Geometry: final body of the model. Coordinates: model frame, mm. A direction names the side the tool comes from. Round coordinates to 2 decimals unless told otherwise and drop trailing zeros. Loops run counter-clockwise (first coordinate to the right, second up) from the corner with the lowest first, then second, coordinate; pieces in that order, holes last. Notation, with made-up numbers: M 50,-1 L 69,-1 A32 ccw 69,26 Z; hole C 39.25,-18 d11. An arc over 180 degrees is marked long. Answer as a JSON object with one key per item and string values.
from build123d import *

# Parameters (mm, degrees)
AUFSATZ_LINEAR_AUSTRAGEN1_DEPTH = 50
SKIZZE2_R                       = 87.5
SKIZZE2_R_2                     = 35
AUFSATZ_LINEAR_AUSTRAGEN2_DEPTH = 50
SCHNITT_LINEAR_AUSTRAGEN1_DEPTH = 50


with BuildPart() as part:
    # Skizze1 → Aufsatz-Linear austragen1 (new body)
    with BuildSketch(Plane.XY):
        Polygon((0, 2300), (50, 2300), (475, 1237.5), (900, 2300), (950, 2300), (950, 2250), (510, 1150), (950, 50), (950, 0), (900, 0), (475, 1062.5), (50, 0), (0, 0), (0, 50), (440, 1150), (0, 2250), align=None)
    extrude(amount=AUFSATZ_LINEAR_AUSTRAGEN1_DEPTH)

    # Skizze2 → Aufsatz-Linear austragen2 (add)
    with BuildSketch(Plane.XY.offset(50)):
        with Locations((475, 1150)):
            Circle(SKIZZE2_R)
        with Locations((475, 1150)):
            Circle(SKIZZE2_R_2, mode=Mode.SUBTRACT)
    extrude(amount=-AUFSATZ_LINEAR_AUSTRAGEN2_DEPTH)

    # Skizze4 → Schnitt-Linear austragen1 (cut)
    with BuildSketch(Plane.XY.offset(50)):
        with BuildLine():
            ThreePointArc((512.5, 1150), (501.516504294, 1176.516504294), (475, 1187.5))
            Line((475, 1187.5), (475, 1112.5))
            ThreePointArc((475, 1112.5), (501.516504294, 1123.483495706), (512.5, 1150))
        make_face()
        with BuildLine():
            Line((475, 1112.5), (475, 1187.5))
            ThreePointArc((475, 1187.5), (437.5, 1150), (475, 1112.5))
        make_face()
    extrude(amount=-SCHNITT_LINEAR_AUSTRAGEN1_DEPTH, mode=Mode.SUBTRACT)


solid = part.part
1) Pin query (flat end, axial travel): P1, Ø1.5, axis at x = 240.5, z = 32.5, coming from the -Y side (3 decimals); P2, Ø5, axis at y = 467, z = 22.5, coming from the -X side; P3, Ø8, axis at y = 1826.5, z = 26, coming from the -X side. Return the tip coordinate at first contact, or that it passes through.
Results:
{"P1": "y = 474.375", "P2": "x = 165.8", "P3": "x = 167.8"}
2) Section query C-C (z = 26). Return the cut outline in (x, y), and give its area (3 significant figures).
Results:
{"outline": "M 0,0 L 50,0 L 475,1062.5 L 900,0 L 950,0 L 950,50 L 535.34,1086.64 A87.5 ccw 535.34,1213.36 L 950,2250 L 950,2300 L 900,2300 L 475,1237.5 L 50,2300 L 0,2300 L 0,2250 L 414.66,1213.36 A87.5 ccw 414.66,1086.64 L 0,50 Z; hole C 475,1150 d75", "area": "317,000 mm2"}
3) Reachability of faces 4 (the flat face through (745.575, 1738.937, 24.65)), 5 (the flat face through (690.475, 523.813, 24.65)), 6 (the flat face through (204.425, 561.063, 24.65)), 7 (the flat face through (950, 2275, 25)), 8 (the flat face through (437.6, 1155.4, 0)) from +Z, -Z, +X, -X, +Y, -Y: full face, straight path, thin tool, end or side. Return the list, or none.
Results:
{"face 4": "+Z, -Z, +X", "face 5": "+Z, -Z, -Y", "face 6": "+Z, -Z, -X", "face 7": "+Z, -Z, +X, +Y, -Y", "face 8": "-Z, +X, -X, +Y, -Y"}
4) Section query A-A (x = 824.5). Return the cut outline in (y, z).
Results:
{"outline": "M 188.75,0 L 363.75,0 L 363.75,50 L 188.75,50 Z; M 1936.25,0 L 2111.25,0 L 2111.25,50 L 1936.25,50 Z"}
5) Section query B-B (y = 316.5). Return the cut outline in (x, z).
Results:
{"outline": "M 106.6,0 L 176.6,0 L 176.6,50 L 106.6,50 Z; M 773.4,0 L 843.4,0 L 843.4,50 L 773.4,50 Z"}
6) Pull-direction query (Y, two-part tool) for faces 1 (the flat face through (437.6, 1155.4, 50)), 2 (the flat face through (25, 2300, 25)), 3 (the flat face through (210.23, 1724.42, 24.65)); classes: +Y half, -Y half, draft (parallel to the pull), parting line (faces both ways), or undercut.
Results:
{"face 1": "draft", "face 2": "+Y half", "face 3": "undercut"}
7) Ray query, line 1 (X direction, y = 1953.5, z = 26.5); line 2 (X direction, y = 1163.5, z = 33); line 3 (Y direction, x = 777.5, z = 43.5). Return the intervals inside material, ascending.
Results:
{"line 1": "118.6 to 188.6, 761.4 to 831.4", "line 2": "388.55 to 440.01, 509.99 to 561.45", "line 3": "306.25 to 481.25, 1818.75 to 1993.75"}
